Geometry: see drawing. Coordinates: mm, zero at the bounding-box minimum. A direction names the side the tool comes from. Round coordinates to 2 decimals unless told otherwise and drop trailing zeros. Loops run counter-clockwise (first coordinate to the right, second up) from the corner with the lowest first, then second, coordinate; pieces in that order, holes last.
(1) Set-up query: the marked faces 1, 2 and 3. Return all of +Z, -Z, +X, -X, +Y, -Y with unobstructed straight access to the full face (end or side cutting, diameter ignored); none if empty.
(2) Material intervals for probe 1 along Z at (x, y) = (20, 20) (3 decimals); probe 2 along Y at (x, z) = (7.95, 35.8) (3 decimals); probe 3 along Y at (x, z) = (15, 28.5), sorted ascending.
(3) First-contact query: pin 1 Ø3 at (y, z) = (21, 16.5) entering from +X; pin 2 Ø10 at (x, z) = (42.5, 5) entering from -Y; pin 3 Ø6 at (x, z) = (35.5, 26.5) entering from +Y; pin 4 Ø1.2 at (x, z) = (20, 27.675) entering from -Y. Flat tips, straight axial feed; report the tip coordinate or a pass-through.
(4) Section B-B, the plane z = 5.5. Return the cut outline in (x, y).
(5) Section D-D, the plane x = 25. Return the cut outline in (y, z), plus the area to 3 significant figures.
(6) Section C-C, the plane y = 7.11. Return the cut outline in (x, z) (3 decimals).
(7) Section A-A, the plane x = 43. Return the cut outline in (y, z) (3 decimals).
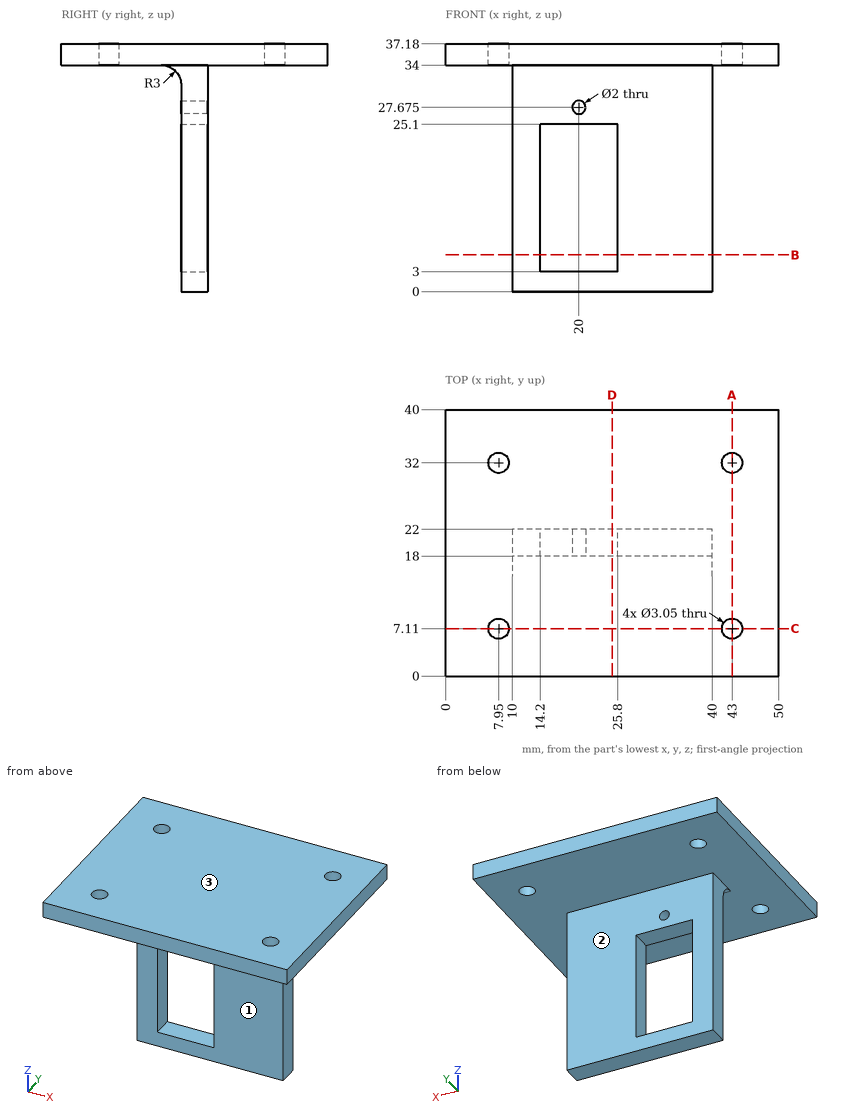
Output values:
1. face 1: -Z, +X, -X, -Y
1. face 2: -Z, +X, -X, +Y
1. face 3: +Z, +X, -X, +Y, -Y
2. probe 1: z = 0 to 3, 25.1 to 26.675, 28.675 to 37.18
2. probe 2: y = 0 to 5.585, 8.635 to 30.475, 33.525 to 40
2. probe 3: y = 18 to 22
3. pin 1: stops at x = 40
3. pin 2: stops at y = 18
3. pin 3: stops at y = 22
3. pin 4: passes through
4. outline: (10, 18) - (14.2, 18) - (14.2, 22) - (10, 22) - close; (25.8, 18) - (40, 18) - (40, 22) - (25.8, 22) - close
5. outline: (0, 34) - (15, 34) arc R3 cw to (18, 31) - (18, 25.1) - (22, 25.1) - (22, 34) - (40, 34) - (40, 37.18) - (0, 37.18) - close; (18, 0) - (22, 0) - (22, 3) - (18, 3) - close
5. area: 177 mm2
6. outline: (0, 34) - (6.425, 34) - (6.425, 37.18) - (0, 37.18) - close; (9.475, 34) - (41.475, 34) - (41.475, 37.18) - (9.475, 37.18) - close; (44.525, 34) - (50, 34) - (50, 37.18) - (44.525, 37.18) - close
7. outline: (0, 34) - (5.585, 34) - (5.585, 37.18) - (0, 37.18) - close; (8.635, 34) - (30.475, 34) - (30.475, 37.18) - (8.635, 37.18) - close; (33.525, 34) - (40, 34) - (40, 37.18) - (33.525, 37.18) - close
